Source: CAD feature listing. Evaluate the final solid. Frame: model axes, mm. A direction names the side the tool comes from. Round coordinates to 2 decimals unless told otherwise and drop trailing zeros. Loops run counter-clockwise (first coordinate to the right, second up) from the corner with the lowest first, then second, coordinate; pieces in that order, holes last.
(1) First-contact query: pin 1 Ø5 at (x, z) = (40, 16.5) entering from +Y. Flat tip, straight axial feed; report the tip coordinate or a pass-through.
(2) Section B-B, the plane x = -47. Return the cut outline in (y, z), plus the area to 3 significant figures.
(3) Section D-D, the plane z = -20. Return the cut outline in (x, y).
(4) Mould query, pull axis X, two halves, no side actions, for faces 1 (the flat face through (55, 90, -20)), 2 (the flat face through (-60, 44, 6)), 3 (the flat face through (45, 5, -15)). Classes: pulls with the +X half, pulls with the -X half, needs draft (parallel to the pull), parting line crosses it, or undercut.
(5) Section C-C, the plane z = -10.5. Return the cut outline in (x, y).
(6) Material intervals for probe 1 along X at (y, z) = (38, 16.5); probe 2 along X at (y, z) = (8.5, -9); probe 3 along X at (y, z) = (45, 11), sorted ascending.
(7) Set-up query: faces 4 (the flat face through (55, 49, -15)), 5 (the flat face through (-50, 49, -20)), 6 (the flat face through (40, 5, -20)), 7 (the flat face through (50, 5, 0)). Return all of +Z, -Z, +X, -X, +Y, -Y with unobstructed straight access to the full face (end or side cutting, diameter ignored); none if empty.
(8) Section A-A, the plane y = 30. Return the cut outline in (x, z), plus the area to 3 significant figures.
```python
from build123d import *

# Parameters (mm, degrees)
SKETCH_1_W          = 120
SKETCH_1_H          = 50
SKETCH_1_W_2        = 100
SKETCH_1_H_2        = 30
EXTRUDE_1_DEPTH     = 10
SKETCH_2_W          = 5
SKETCH_2_H          = 20
SKETCH_2_W_2        = 10
SKETCH_2_H_2        = 10
SKETCH_2_W_3        = 3
EXTRUDE_2_DEPTH     = 80
SKETCH_3_W          = 55
SKETCH_3_H          = 10
CUT_EXTRUDE_1_DEPTH = 112.018016556


with BuildPart() as part:
    # 草图1 → 凸台-拉伸1 (new body)
    with BuildSketch(Plane(origin=(0, 0, 0), x_dir=(1, 0, 0), z_dir=(0, 1, 0))):
        Rectangle(SKETCH_1_W, SKETCH_1_H)
        Rectangle(SKETCH_1_W_2, SKETCH_1_H_2, mode=Mode.SUBTRACT)
    extrude(amount=EXTRUDE_1_DEPTH)

    # 草图2 → 凸台-拉伸2 (add)
    with BuildSketch(Plane(origin=(0, 10, 0), x_dir=(1, 0, 0), z_dir=(0, 1, 0))):
        with Locations((57.5, -15)):
            Rectangle(SKETCH_2_W, SKETCH_2_H)
        with Locations((-57.5, -15)):
            Rectangle(SKETCH_2_W, SKETCH_2_H)
        with Locations((-55, 20)):
            Rectangle(SKETCH_2_W_2, SKETCH_2_H_2)
        with Locations((55, 20)):
            Rectangle(SKETCH_2_W_2, SKETCH_2_H_2)
        with Locations((-40.5, -20)):
            Rectangle(SKETCH_2_W_3, SKETCH_2_H_2)
    extrude(amount=EXTRUDE_2_DEPTH)

    # 草图3 → 切除-拉伸1 (cut, through all)
    with BuildSketch(Plane.XZ):
        with Locations((12.5, -20)):
            Rectangle(SKETCH_3_W, SKETCH_3_H)
    extrude(amount=-CUT_EXTRUDE_1_DEPTH, mode=Mode.SUBTRACT)


solid = part.part
```
Output values:
1. pin 1: stops at y = 10
2. outline: (0, -25) - (10, -25) - (10, -15) - (0, -15) - close; (0, 15) - (10, 15) - (10, 25) - (0, 25) - close
2. area: 200 mm2
3. outline: (-60, 0) - (-15, 0) - (-15, 10) - (-50, 10) - (-50, 90) - (-60, 90) - close; (40, 0) - (60, 0) - (60, 90) - (50, 90) - (50, 10) - (40, 10) - close
4. face 1: needs draft
4. face 2: pulls with the -X half
4. face 3: undercut
5. outline: (-60, 0) - (-50, 0) - (-50, 10) - (-60, 10) - close; (50, 0) - (60, 0) - (60, 10) - (50, 10) - close
6. probe 1: x = -60 to -55, -42 to -39, 55 to 60
6. probe 2: x = -60 to -50, 50 to 60
6. probe 3: x = -60 to -55, 55 to 60
7. face 4: +X, -X, +Y
7. face 5: +Z, -Z, +Y
7. face 6: -Z, +Y, -Y
7. face 7: +Y, -Y
8. outline: (-60, -25) - (-50, -25) - (-50, -15) - (-60, -15) - close; (-60, 5) - (-55, 5) - (-55, 25) - (-60, 25) - close; (-42, 15) - (-39, 15) - (-39, 25) - (-42, 25) - close; (50, -25) - (60, -25) - (60, -15) - (50, -15) - close; (55, 5) - (60, 5) - (60, 25) - (55, 25) - close
8. area: 430 mm2
